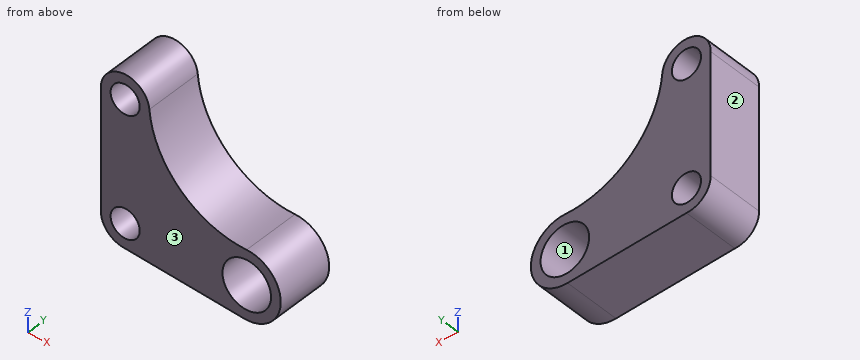
```python
from build123d import *

# Parameters (mm, degrees)
F0_R     = 3
F0_R_2   = 5
F1_DEPTH = 12


with BuildPart() as f1:
    # F0 (on Front) → F1 (new body)
    with BuildSketch(Plane.XZ):
        with BuildLine():
            Line((-5, 24.77), (-5, 0))
            ThreePointArc((-5, 0), (-3.535534, -3.535534), (0, -5))
            Line((0, -5), (24.455898, -6.977234))
            ThreePointArc((24.455898, -6.977234), (32.014914, -0.266785), (24.988984, 6.999931))
            ThreePointArc((24.988984, 6.999931), (11.436354, 12.210538), (4.980073, 25.215947))
            ThreePointArc((4.980073, 25.215947), (-0.223196, 29.765016), (-5, 24.77))
        make_face()
        Circle(F0_R, mode=Mode.SUBTRACT)
        with Locations((25.02, 0)):
            Circle(F0_R_2, mode=Mode.SUBTRACT)
        with Locations((0, 24.77)):
            Circle(F0_R, mode=Mode.SUBTRACT)
    extrude(amount=F1_DEPTH)


solid = f1.part
```
For this review, take the finished solid that the model builds, in its own axes (mm). Face numbers are marked on the shaded views. Round coordinates to 2 decimals unless told otherwise and drop trailing zeros. Write each loop counter-clockwise with the first axis right and the second up, starting at its lowest first coordinate (ties: lowest second). Pieces come first, ordered by that corner, then holes. Notation, with made-up numbers: (77, -6.5) - (101, -6.5) arc R29 ccw to (101, 32.5) - close; hole circle Ø2 at (-28, -20.5). An arc over 180 degrees is marked (long way). Answer as CSV lines item,"result". Start each with the question number.
(1) Add section C-C, the plane y = -9.25. State the section outline as (x, z) points.
(2) For line 1 (Z direction, x = 0, y = -4); line 2 (Z direction, x = 25.02, y = -7); line 3 (Z direction, x = -2.5, y = -6.5), list the stretches that pass through material, from the lowest coordinate up.
(3) Add section D-D, the plane x = 24. State the section outline as (y, z) points.
(4) Add section A-A, the plane z = -4. State the section outline as (x, y) points, plus the area to 3 significant figures.
(5) For pin 1 (4 mm diameter, centred on x = 28, y = -1.5, fed in from -Z); pin 2 (2 mm diameter, centred on x = -0.5, y = -9, fed in from +Z), all flat-tipped, find the tip position at first contact; note any pin that passes through.
(6) Mouldability with a two-part tool opening along X and no side actions: class the marked faces 1, 2 and 3 as +X half, -X half, draft (parallel to the pull), parting line (faces both ways), or undercut.
(7) Add section B-B, the plane x = -0.5. State the section outline as (y, z) points.
From the geometry:
1,outline,"(-5, 0) arc R5 ccw to (0, -5) - (24.46, -6.98) arc R7 ccw (long way) to (24.99, 7) arc R20 cw to (4.98, 25.22) arc R5 ccw to (-5, 24.77) - close; hole circle Ø6 at (0, 0); hole circle Ø6 at (0, 24.77); hole circle Ø10 at (25.02, 0)"
2,line 1,"z = -5 to -3, 3 to 21.77, 27.77 to 29.77"
2,line 2,"z = -7 to -5, 5 to 7"
2,line 3,"z = -4.33 to -1.66, 1.66 to 23.11, 26.43 to 29.1"
3,outline,"(-12, -6.94) - (0, -6.94) - (0, -4.89) - (-12, -4.89) - close; (-12, 4.89) - (0, 4.89) - (0, 7.02) - (-12, 7.02) - close"
4,outline,"(-3, -12) - (22.02, -12) - (22.02, 0) - (-3, 0) - close; (28.02, -12) - (30.76, -12) - (30.76, 0) - (28.02, 0) - close"
4,area,"333 mm²"
5,pin 1,"stops at z = -6.93"
5,pin 2,"stops at z = 29.77"
6,face 1,"undercut"
6,face 2,"-X half"
6,face 3,"draft"
7,outline,"(-12, -4.97) - (0, -4.97) - (0, -2.96) - (-12, -2.96) - close; (-12, 2.96) - (0, 2.96) - (0, 21.81) - (-12, 21.81) - close; (-12, 27.73) - (0, 27.73) - (0, 29.74) - (-12, 29.74) - close"
